from build123d import *

# Parameters (mm, degrees)
SKETCH1_R           = 5
SKETCH1_R_2         = 2.7
BOSS_EXTRUDE1_DEPTH = 15.5
BOSS_EXTRUDE2_START = 15.5
SKETCH1_4_R         = 2.7
BOSS_EXTRUDE2_DEPTH = 4
FILLET1_R           = 0.5


with BuildPart() as part:
    # Sketch1 → Boss-Extrude1 (new body)
    # profile 1 of 2: a face of its own
    with BuildSketch(Plane(origin=(0, 0, 0), x_dir=(1, 0, 0), z_dir=(0, 1, 0))):
        with Locations(Location((0, 0, 0), (0, 0, 270))):
            Circle(SKETCH1_R)
        Circle(SKETCH1_R_2, mode=Mode.SUBTRACT)
    # profile 2 of 2: a face of its own
    with BuildSketch(Plane(origin=(0, 0, 0), x_dir=(1, 0, 0), z_dir=(0, 1, 0))):
        Circle(SKETCH1_R_2)
    extrude(amount=BOSS_EXTRUDE1_DEPTH)

    # Sketch1<4> → Boss-Extrude2 (add)
    with BuildSketch(Plane(origin=(0, 0, 0), x_dir=(1, 0, 0), z_dir=(0, 1, 0)).offset(BOSS_EXTRUDE2_START)):
        with Locations(Location((0, 0, 0), (0, 0, 270))):
            Circle(SKETCH1_4_R)
    extrude(amount=BOSS_EXTRUDE2_DEPTH)

    # Fillet1
    fillet1_edges = [part.edges().sort_by_distance(p)[0] for p in [
        (0, 15.5, -2.7),
    ]]
    fillet(fillet1_edges, radius=FILLET1_R)


solid = part.part
The model under review builds one solid part; all positions refer to its coordinate system, in mm. A direction names the side the tool comes from. Coordinates: 2 decimals unless noted, no trailing zeros. Write each loop counter-clockwise with the first axis right and the second up, starting at its lowest first coordinate (ties: lowest second). Pieces come first, ordered by that corner, then holes. Notation, with made-up numbers: (26, 31.5) - (46, 31.5) arc R15 cw to (46, 57.5) - close; hole circle Ø5 at (-10, -36.75). An arc over 180 degrees is marked (long way). Answer as a JSON object with one key per item and string values. Group by question number.
1. Clearance check with flat-ended pins moving along their axes: pin 1 Ø2 at (y, z) = (12.5, 3) entering from -X; pin 2 Ø5 at (y, z) = (10.5, -3.5) entering from +X; pin 3 Ø1 at (y, z) = (14.5, 3.5) entering from -X. State where each tip first meets the part, or that it passes through.
2. Add section B-B (z = 0). Give the boundary of the cut face in (x, y).
3. Add section A-A (x = 0). Give the boundary of the cut face in (y, z), plus the area to 3 significant figures.
4. Add section D-D (z = 3.75). Give the boundary of the cut face in (x, y), plus the area to 3 significant figures.
5. Add section C-C (y = 10.75). Give the boundary of the cut face in (x, z), plus the area to 3 significant figures.
6. Machinability: for faces 1 (the face through (0, 0, 0)), 2 (the face through (-1, 15.5, 3.3)), which of the approach directions +Z, -Z, +X, -X, +Y, -Y give a long, thin tool a straight path to every point of the face, cutting with its end or side? Answer none if there is none.
7. To check wall thickness, follow probe 1 along Y at (x, z) = (-1, -3); probe 2 along X at (y, z) = (18.5, 2.25); probe 3 along X at (y, z) = (8.75, -0.5). State the ranges of each line that lie inside material, in increasing order.
Findings:
{
 "1": {"pin 1": "x = -4.58", "pin 2": "x = 4.9", "pin 3": "x = -4"},
 "2": {"outline": "(-5, 0) - (5, 0) - (5, 15.5) - (3.2, 15.5) arc R0.5 cw to (2.7, 16) - (2.7, 19.5) - (-2.7, 19.5) - (-2.7, 16) arc R0.5 cw to (-3.2, 15.5) - (-5, 15.5) - close"},
 "3": {"outline": "(0, -5) - (15.5, -5) - (15.5, -3.2) arc R0.5 cw to (16, -2.7) - (19.5, -2.7) - (19.5, 2.7) - (16, 2.7) arc R0.5 cw to (15.5, 3.2) - (15.5, 5) - (0, 5) - close", "area": "177 mm²"},
 "4": {"outline": "(-3.31, 0) - (3.31, 0) - (3.31, 15.5) - (-3.31, 15.5) - close", "area": "103 mm²"},
 "5": {"outline": "circle Ø10 at (0, 0)", "area": "78.5 mm²"},
 "6": {"face 1": "+Z, -Z, +X, -X, -Y", "face 2": "+Y"},
 "7": {"probe 1": "0 to 15.5", "probe 2": "-1.49 to 1.49", "probe 3": "-4.97 to 4.97"}
}
